For this review, take the finished solid that the model builds, in its own axes (mm). A direction names the side the tool comes from. Give positions to 0.01 mm unless a question says otherwise; leave off trailing zeros. Write each loop counter-clockwise with the first axis right and the second up, starting at its lowest first coordinate (ties: lowest second). Pieces come first, ordered by that corner, then holes. Notation, with made-up numbers: M -14.5,82.25 L 27.5,82.25 A27 cw 27.5,102.25 Z; hole C -19,-10 d10. An arc over 180 degrees is marked long. Answer as a JSON object with one key per item and string values. Group by question number.
```python
from build123d import *

# Parameters (mm, degrees)
SKETCH4_R           = 68.072
BOSS_EXTRUDE2_DEPTH = 0.508
SKETCH5_R           = 55.372
CUT_EXTRUDE5_DEPTH  = 1.508
CUT_EXTRUDE6_DEPTH  = 1.508
CUT_EXTRUDE11_DEPTH = 1.508


with BuildPart() as part:
    # Sketch4 → Boss-Extrude2 (new body)
    with BuildSketch(Plane.XY):
        Circle(SKETCH4_R)
    extrude(amount=BOSS_EXTRUDE2_DEPTH)

    # Sketch5 → Cut-Extrude5 (cut, through all)
    with BuildSketch(Plane.XY.offset(0.508)):
        Circle(SKETCH5_R)
    extrude(amount=-CUT_EXTRUDE5_DEPTH, mode=Mode.SUBTRACT)

    # Sketch6 → Cut-Extrude6 (cut, through all)
    with BuildSketch(Plane.XY.offset(0.508)):
        with BuildLine():
            ThreePointArc((46.966739661, 46.966739366), (40.321349994, 46.966739524), (40.32135011, 40.321349857))
            ThreePointArc((40.32135011, 40.321349857), (52.682382823, 21.821756782), (57.023, -1.08e-06))
            ThreePointArc((57.023, -1.08e-06), (61.721999911, -4.699), (66.421, -1.258e-06))
            ThreePointArc((66.421, -1.258e-06), (61.36500271, 25.418215583), (46.966739661, 46.966739366))
        make_face()
        with BuildLine():
            ThreePointArc((46.966739366, -46.966739661), (46.966739524, -40.321349994), (40.321349857, -40.32135011))
            ThreePointArc((40.321349857, -40.32135011), (21.821756782, -52.682382823), (-1.08e-06, -57.023))
            ThreePointArc((-1.08e-06, -57.023), (-4.699, -61.721999911), (-1.258e-06, -66.421))
            ThreePointArc((-1.258e-06, -66.421), (25.418215583, -61.36500271), (46.966739366, -46.966739661))
        make_face()
        with BuildLine():
            ThreePointArc((-46.966739661, -46.966739366), (-40.321349994, -46.966739524), (-40.32135011, -40.321349857))
            ThreePointArc((-40.32135011, -40.321349857), (-52.682382823, -21.821756782), (-57.023, 1.08e-06))
            ThreePointArc((-57.023, 1.08e-06), (-61.721999911, 4.699), (-66.421, 1.258e-06))
            ThreePointArc((-66.421, 1.258e-06), (-61.36500271, -25.418215583), (-46.966739661, -46.966739366))
        make_face()
        with BuildLine():
            ThreePointArc((-46.966739366, 46.966739661), (-46.966739524, 40.321349994), (-40.321349857, 40.32135011))
            ThreePointArc((-40.321349857, 40.32135011), (-21.821756782, 52.682382823), (1.08e-06, 57.023))
            ThreePointArc((1.08e-06, 57.023), (4.699, 61.721999911), (1.258e-06, 66.421))
            ThreePointArc((1.258e-06, 66.421), (-25.418215583, 61.36500271), (-46.966739366, 46.966739661))
        make_face()
    extrude(amount=-CUT_EXTRUDE6_DEPTH, mode=Mode.SUBTRACT)

    # Sketch8 → Cut-Extrude11 (cut, through all)
    with BuildSketch(Plane.XY.offset(0.508)):
        Polygon((63.962998999, 25.119703581), (62.990983081, 27.466357594), (61.817656075, 26.980349635), (62.789671993, 24.633695622), align=None)
        Polygon((-25.119703581, 63.962998999), (-27.466357594, 62.990983081), (-26.980349635, 61.817656075), (-24.633695622, 62.789671993), align=None)
        Polygon((-62.990983081, 27.466357594), (-63.962998999, 25.119703581), (-62.789671993, 24.633695622), (-61.817656075, 26.980349635), align=None)
        Polygon((-63.962998999, -25.119703581), (-62.990983081, -27.466357594), (-61.817656075, -26.980349635), (-62.789671993, -24.633695622), align=None)
        Polygon((-27.466357594, -62.990983081), (-25.119703581, -63.962998999), (-24.633695622, -62.789671993), (-26.980349635, -61.817656075), align=None)
        Polygon((25.119703581, -63.962998999), (27.466357594, -62.990983081), (26.980349635, -61.817656075), (24.633695622, -62.789671993), align=None)
        Polygon((62.990983081, -27.466357594), (63.962998999, -25.119703581), (62.789671993, -24.633695622), (61.817656075, -26.980349635), align=None)
        Polygon((27.466357594, 62.990983081), (25.119703581, 63.962998999), (24.633695622, 62.789671993), (26.980349635, 61.817656075), align=None)
    extrude(amount=-CUT_EXTRUDE11_DEPTH, mode=Mode.SUBTRACT)


solid = part.part
```
Item 1: To check wall thickness, follow probe 1 along X at (y, z) = (-2.5, 0.35); probe 2 along Y at (x, z) = (23.5, 0.05); probe 3 along Y at (x, z) = (12.5, 0.25). State the ranges of each line that lie inside material, in increasing order.
Item 2: Consider section B-B (y = 11). Give the boundary of the cut face in (x, z).
Item 3: Draft analysis for pull direction Y (two halves, no side actions). For faces 1 (the cylindrical face through (48.386, 47.881, 0.25)), 2 (the cylindrical face through (22.11, -52.56, 0.26)), 3 (the cylindrical face through (68.07, -0.36, 0.25)), state which applies: released by +Y, released by -Y, zero draft, split by the parting line, or undercut.
Item 4: Consider section C-C (z = 0.3). State how many separate pieces and enclosed holes the cut face has, plus the area to 3 significant figures.
Item 5: Machinability: for faces 4 (the cylindrical face through (4.698, 61.619, 0.258)), 5 (the flat face through (0, 56, 0.508)), which of the approach directions +Z, -Z, +X, -X, +Y, -Y give a long, thin tool a straight path to every point of the face, cutting with its end or side? Answer none if there is none.
Item 6: Consider section D-D (y = -42). Give the boundary of the cut face in (x, z).
Item 7: Consider section A-A (x = -34). Give the boundary of the cut face in (y, z), plus the area to 3 significant figures.
Result set:
{
 "1": {"probe 1": "x = -68.03 to -66.37, -56.97 to -55.32, 55.32 to 57.74, 65.7 to 68.03", "probe 2": "y = -63.89 to -62.12, -51.96 to -50.14, 50.14 to 63.89", "probe 3": "y = -66.91 to -65.23, -55.64 to -53.94, 53.94 to 66.91"},
 "2": {"outline": "M -67.18,0 L -54.27,0 L -54.27,0.51 L -67.18,0.51 Z; M 54.27,0 L 55.95,0 L 55.95,0.51 L 54.27,0.51 Z; M 65.5,0 L 67.18,0 L 67.18,0.51 L 65.5,0.51 Z"},
 "3": {"face 1": "released by +Y", "face 2": "undercut", "face 3": "split by the parting line"},
 "4": {"separate pieces": "1", "enclosed holes": "5", "area": "2,810 mm^2"},
 "5": {"face 4": "+Z, -Z", "face 5": "+Z, +X, -X, +Y, -Y"},
 "6": {"outline": "M -53.57,0 L -51.46,0 L -51.46,0.51 L -53.57,0.51 Z; M -39.24,0 L -36.08,0 L -36.08,0.51 L -39.24,0.51 Z; M 36.08,0 L 38.57,0 L 38.57,0.51 L 36.08,0.51 Z; M 48.05,0 L 53.57,0 L 53.57,0.51 L 48.05,0.51 Z"},
 "7": {"outline": "M -58.97,0 L -43.7,0 L -43.7,0.51 L -58.97,0.51 Z; M 43.7,0 L 45.78,0 L 45.78,0.51 L 43.7,0.51 Z; M 57.06,0 L 58.97,0 L 58.97,0.51 L 57.06,0.51 Z", "area": "9.78 mm^2"}
}
